Here's how the part is built. I have some questions about the finished solid (model axes, mm). A direction names the side the tool comes from. Round coordinates to 2 decimals unless told otherwise and drop trailing zeros. Loops run counter-clockwise (first coordinate to the right, second up) from the corner with the lowest first, then second, coordinate; pieces in that order, holes last. Notation, with made-up numbers: M -27.75,84.25 L -17.75,84.25 A14 cw -17.75,94.25 Z; hole C 47,24.5 d8. An arc over 180 degrees is marked long. Use a Markdown table: item, result.
Autodesk Inventor part; units mm, degrees
ref_plane "YZ Plane" through (0, 0, 0) normal (1, 0, 0) x (0, 1, 0)
ref_plane "XZ Plane" through (0, 0, 0) normal (0, 1, 0) x (-1, 0, 0)
ref_plane "XY Plane" through (0, 0, 0) normal (0, 0, 1) x (1, 0, 0)
sketch "Sketch1" plane through (0, 0, 0) normal (0, 1, 0) x (-1, 0, 0)
  line L0 (0, 0) -> (-38.1, 0)
  line L1 (-38.1, 0) -> (-38.1, -76.2)
  line L2 (-38.1, -76.2) -> (0, -76.2)
  line L3 (0, -76.2) -> (0, 0)
  dimension "d0" = 38.1
  dimension "d1" = 76.2
extrude "Extrusion1" add sketch "Sketch1" along normal blind 2.54
sketch "Sketch2" plane through (0, 2.54, 0) normal (0, 1, 0) x (1, 0, 0)
  line L0 (38.1, 76.2) -> (0, 76.2)
  line L1 (0, 76.2) -> (38.1, 76.2)
  line L2 (38.1, 76.2) -> (38.1, 63.5)
  line L3 (38.1, 63.5) -> (0, 63.5)
  line L4 (0, 63.5) -> (0, 76.2)
  point P0 (0, 0)
  dimension "d4" = 38.1
  dimension "d5" = 12.7
extrude "Extrusion2" add sketch "Sketch2" along normal blind 25.4
sketch "Sketch6" plane through (0, 27.94, 0) normal (0, 1, 0) x (1, 0, 0)
  line L0 (0, 76.2) -> (0, 63.5)
  line L1 (0, 69.85) -> (38.1, 69.85)
  line L2 (38.1, 63.5) -> (38.1, 76.2)
  line L3 (0, 69.85) -> (9.525, 69.85)
  line L4 (38.1, 69.85) -> (28.575, 69.85)
  point P0 (0, 0)
  dimension "d8" = 9.525
  dimension "d9" = 9.525
hole "Hole1" at (9.525, 27.94, -69.85) at (28.575, 27.94, -69.85) direction (0, -1, 0) diameter 5.08 depth 12.7 tip angle 118
sketch "Sketch7" plane through (0, 0, 0) normal (0, -1, 0) x (1, 0, 0)
  line L0 (38.1, 0) -> (38.1, -76.2)
  line L1 (38.1, -38.1) -> (27.94, -38.1)
  line L2 (38.1, -76.2) -> (0, -76.2)
  line L3 (19.05, -76.2) -> (19.05, -71.12)
  line L4 (0, 0) -> (38.1, 0)
  line L5 (19.05, 0) -> (19.05, -5.08)
  line L6 (19.05, -71.12) -> (38.1, -71.12)
  line L7 (27.94, -38.1) -> (27.94, -71.12)
  line L8 (27.94, -71.12) -> (-13.208, -71.12)
  line L9 (-13.208, -71.12) -> (-13.208, -5.08)
  line L10 (-13.208, -5.08) -> (27.94, -5.08)
  line L11 (27.94, -5.08) -> (27.94, -71.12)
  dimension "d23" = 10.16
  dimension "d24" = 5.08
  dimension "d25" = 5.08
  dimension "d26" = 41.148
extrude "Extrusion3" add sketch "Sketch7" along normal blind 14.224 contours L7 L6 L8 L9 L10 L11
chamfer "Chamfer3" distance 41.148 distance2 14.224 1 edges at (27.94, -14.224, -38.1) measured on face at (14.224, -14.224, -49.1067)
properties part number "Base"
1. I need wall thicknesses on probe 1 along X at (y, z) = (25, -69.85) (3 decimals); probe 2 along X at (y, z) = (24, -69); probe 3 along Z at (x, y) = (16.5, 26.5). Which ranges of each line are inside material? Lowest first, please. Write a range as from..to.
Answer sheet:
| item | result |
|---|---|
| probe 1 | 0..6.985, 12.065..26.035, 31.115..38.1 |
| probe 2 | 0..7.13, 11.92..26.18, 30.97..38.1 |
| probe 3 | -76.2..-63.5 |
2. Which directions (+Z, -Z, +X, -X, +Y, -Y) give clear straight access to the entire face, cutting with the end or side of a thin tool? Please do faces 4 (the face through (-7, 0, -38)), 5 (the face through (3, -5, -71.12)), 6 (the face through (19, 2.54, -31)).
Answer sheet:
| item | result |
|---|---|
| face 4 | +Z, -Z, -X, +Y |
| face 5 | -Z, +X, -X, -Y |
| face 6 | +Z, +X, -X, +Y |
3. We'd pull the mould along X, two halves only. Please class faces 1 (the face through (0, 10, -64)), 2 (the face through (28.71, 13.98, -69.43)), 3 (the face through (32, 0, -38)): +X half, -X half, draft (parallel to the pull), parting line (faces both ways), or undercut.
Answer sheet:
| item | result |
|---|---|
| face 1 | -X half |
| face 2 | undercut |
| face 3 | draft |
4. Imagine slicing it at C-C, the plane y = 22. Write out the boundary of the cut face in (x, z) (3 decimals), then the cut area to 3 significant figures.
Answer sheet:
| item | result |
|---|---|
| outline | M 0,-76.2 L 38.1,-76.2 L 38.1,-63.5 L 0,-63.5 Z; hole C 9.525,-69.85 d5.08; hole C 28.575,-69.85 d5.08 |
| area | 443 mm2 |
5. For pin 1 Ø4 at (x, z) = (5.5, -40) entering from +Y; pin 2 Ø19 at (x, z) = (15, -49) entering from -Y; pin 3 Ø6.5 at (x, z) = (-4.5, -38.5) entering from +Y, each with a flat end and sliding along its axis, tell me the tip position at first contact or that it passes through.
Answer sheet:
| item | result |
|---|---|
| pin 1 | y = 2.54 |
| pin 2 | y = -7.76 |
| pin 3 | y = 0 |
6. Imagine slicing it at D-D, the plane y = 1. Write out the boundary of the cut face in (x, z), then the cut area to 3 significant figures.
Answer sheet:
| item | result |
|---|---|
| outline | M 0,-76.2 L 38.1,-76.2 L 38.1,0 L 0,0 Z |
| area | 2,900 mm2 |
7. Imagine slicing it at B-B, the plane x = 32. Write out the boundary of the cut face in (y, z).
Answer sheet:
| item | result |
|---|---|
| outline | M 0,-76.2 L 27.94,-76.2 L 27.94,-63.5 L 2.54,-63.5 L 2.54,0 L 0,0 Z |
